Verification items for the finished model (mm, model axes). A direction names the side the tool comes from. Round coordinates to 2 decimals unless told otherwise and drop trailing zeros. Write each loop counter-clockwise with the first axis right and the second up, starting at its lowest first coordinate (ties: lowest second). Pieces come first, ordered by that corner, then holes.
Autodesk Inventor part; units mm, degrees
ref_plane "YZ Plane" through (0, 0, 0) normal (1, 0, 0) x (0, 1, 0)
ref_plane "XZ Plane" through (0, 0, 0) normal (0, 1, 0) x (-1, 0, 0)
ref_plane "XY Plane" through (0, 0, 0) normal (0, 0, 1) x (1, 0, 0)
sketch "スケッチ1" plane through (0, 0, 0) normal (1, 0, 0) x (0, 1, 0)
  line L0 (-10, -10) -> (10, -10)
  line L1 (10, -10) -> (10, 10)
  line L2 (10, 10) -> (-10, 10)
  line L3 (-10, 10) -> (-10, -10)
  line L4 (-10, -10) -> (10, 10) construction
  line L5 (10, -10) -> (-10, 10) construction
  point P0 (0, 0)
  dimension "d0" = 20
  dimension "d1" = 20
extrude "プレート1" add sketch "スケッチ1" along normal blind 2
sketch "スケッチ2" plane through (4, 12, 10) normal (0, 1, 0) x (-1, 0, 0)
  line L0 (0, -20) -> (0, 0)
  line L1 (0, 0) -> (-21, 0)
  line L2 (-21, 0) -> (-21, -20)
  line L3 (-21, -20) -> (0, -20)
edge flange "フランジ1" height 25 angle 90 thickness 2 bend radius 2 thickness toward (0, 1, 0) relief straight relief width 2 relief depth 1 edges at (2, 10, 0) wall of the first edge with corners at (4, 12, -10) (4, 12, 10) (25, 12, 10) (25, 12, -10)
bend "曲げ1"
corner "コーナー1"
sketch "スケッチ3" plane through (0, 0, 0) normal (-1, 0, 0) x (0, 0, 1)
  line L0 (-7.5, 6) -> (-7.5, -6)
  arc A0 (-7.5, -6) -> (-4.5, -6) centre (-6, -6) ccw
  line L1 (-4.5, -6) -> (-4.5, 6)
  arc A1 (-4.5, 6) -> (-7.5, 6) centre (-6, 6) ccw
  line L2 (4.5, 6) -> (4.5, -6)
  arc A2 (4.5, -6) -> (7.5, -6) centre (6, -6) ccw
  line L3 (7.5, -6) -> (7.5, 6)
  arc A3 (7.5, 6) -> (4.5, 6) centre (6, 6) ccw
  line L4 (-10, -10) -> (-10, 10)
  line L5 (10, 10) -> (10, -10)
  line L6 (10, -10) -> (-10, -10)
  line L7 (-10, 10) -> (10, 10)
  point P0 (0, 0)
  dimension "d13" = 4
  dimension "d14" = 4
  dimension "d15" = 1.5
  dimension "d16" = 1.5
  dimension "d17" = 4
  dimension "d18" = 4
  dimension "d19" = 4
  dimension "d20" = 4
extrude "押し出し1" cut sketch "スケッチ3" against normal blind 10 contours A1 L1 A0 L0 | A3 L3 A2 L2
equation "\"d2\" = Thickness"
equation "\"d3\" = BendReliefWidth"
equation "\"d4\" = BendReliefDepth"
equation "\"d5\" = MinimumRemnant"
equation "\"d6\" = TransitionRadius"
equation "\"d9\" = BendRadius"
equation "\"d10\" = CornerReliefSize"
equation "\"d11\" = GapSize"
equation "\"d12\" = JacobiRadiusSize"
equation "\"BendRadius\" = Thickness"
equation "\"BendReliefWidth\" = Thickness"
equation "\"BendReliefDepth\" = 0.5 * Thickness"
equation "\"CornerReliefSize\" = 4 * Thickness"
equation "\"MinimumRemnant\" = 2 * Thickness"
equation "\"TransitionRadius\" = BendRadius"
equation "\"JacobiRadiusSize\" = Thickness"
equation "\"GapSize\" = Thickness"
properties part number "trackballL"
Q1. Release check for a two-part mould opening along Y. For faces 1 (the cylindrical face through (1, 7.5, -6)), 2 (the cylindrical face through (1, -7.5, 6)), 3 (the flat face through (0, 0, 0)), 4 (the cylindrical face through (2.6, 11.43, 0.14)) record: released by +Y, released by -Y, zero draft, split by the parting line, or undercut.
Recorded:
face 1: undercut
face 2: undercut
face 3: zero draft
face 4: released by -Y
Q2. Depth check by flat-ended pin: P1, Ø6, axis at y = 4, z = -4, coming from the +X side; P2, Ø4, axis at x = 18, z = -7.5, coming from the -Y side. Enter the tip coordinate at first touch or a pass-through.
Recorded:
P1: stops at x = 2
P2: stops at y = 12
Q3. Sectioned sample at A-A (y = 1.75). Enter the section's corners in (x, z).
Recorded:
outline: (0, -10) - (2, -10) - (2, -7.5) - (0, -7.5) - close; (0, -4.5) - (2, -4.5) - (2, 4.5) - (0, 4.5) - close; (0, 7.5) - (2, 7.5) - (2, 10) - (0, 10) - close
Q4. Sectioned sample at B-B (z = -6). Enter the section's corners in (x, y), plus the area to 3 significant figures.
Recorded:
outline: (0, -10) - (2, -10) - (2, -7.5) - (0, -7.5) - close; (0, 7.5) - (2, 7.5) - (2, 10) arc R2 cw to (4, 12) - (25, 12) - (25, 14) - (4, 14) arc R4 ccw to (0, 10) - close
area: 61.4 mm2
Q5. Material ranges on line 1 along Z through (x, y) = (1.5, -5); line 2 along Y through (x, z) = (4.5, 0.5); line 3 along X through (y, z) = (-8.5, 4.75), recorded low to high.
Recorded:
line 1: z = -10 to -7.5, -4.5 to 4.5, 7.5 to 10
line 2: y = 12 to 14
line 3: x = 0 to 2
Q6. Sectioned sample at D-D (x = 14.25). Enter the section's corners in (y, z).
Recorded:
outline: (12, -10) - (14, -10) - (14, 10) - (12, 10) - close
Q7. Tool access check on faces 5 (the flat face through (2, 0, 0)), 6 (the flat face through (1, 0, 7.5)), 7 (the flat face through (25, 13, 0)). Record the directions out of +Z, -Z, +X, -X, +Y, -Y that give a thin tool (end or side, any length) a straight path to the whole face; none if there is none.
Recorded:
face 5: +Z, -Z, +X, -Y
face 6: +X, -X
face 7: +Z, -Z, +X, +Y, -Y
Q8. Sectioned sample at C-C (z = 2). Enter the section's corners in (x, y).
Recorded:
outline: (0, -10) - (2, -10) - (2, 10) arc R2 cw to (4, 12) - (25, 12) - (25, 14) - (4, 14) arc R4 ccw to (0, 10) - close
